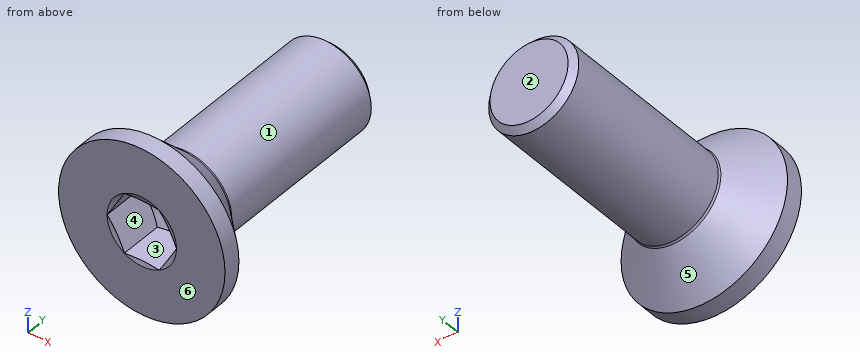
Solid Edge part; units mm, degrees
sketch "Sketch1" plane through (0, 0, 0) normal (0, 0, 1) x (1, 0, 0)
  line L0 (1.5, 0) -> (1.5, 6.14)
  line L1 (0, 6.14) -> (1.5, 6.14)
  line L2 (0, 0) -> (0, 6.14)
  line L3 (0, 0) -> (0, -1.86)
  line L4 (0, -1.86) -> (2.77, -1.86)
  line L5 (2.77, -1.86) -> (2.77, -1.27)
  line L6 (2.77, -1.27) -> (1.5, 0)
revolve "RevolvedProtrusion1" add sketch "Sketch1" angle 360 about axis through (0, 0, 0) along (0, 1, 0)
sketch "Sketch2" plane through (0, 0, 0) normal (1, 0, 0) x (0, 1, 0)
  line L0 (-1.86, 1.6515) -> (-0.76, 1.6515)
  line L1 (0.1935, 0) -> (-0.76, 1.6515)
  line L2 (-1.86, 0) -> (0.1935, 0)
  line L3 (-1.86, 0) -> (-1.86, 1.6515)
revolve "RevolvedCutout1" cut sketch "Sketch2" angle 360 about axis through (0, -4.5, 0) along (0, 1, 0)
sketch "Sketch3" plane through (0, -1.86, 0) normal (0, -1, 0) x (0, 0, 1)
  circle A0 centre (0, 0) radius 1.6515
  line L0 (-1, -0.5774) -> (0, -1.1547)
  line L1 (0, -1.1547) -> (1, -0.5774)
  line L2 (1, -0.5774) -> (1, 0.5774)
  line L3 (1, 0.5774) -> (0, 1.1547)
  line L4 (0, 1.1547) -> (-1, 0.5774)
  line L5 (-1, 0.5774) -> (-1, -0.5774)
extrude "Protrusion1" add sketch "Sketch3" against normal up to next
sketch "Sketch4" plane through (0, 0, 0) normal (0, 0, 1) x (1, 0, 0)
  line L0 (-1.1547, -1.86) -> (0, -1.86)
  line L1 (0, -1.86) -> (0, -1.5506)
  line L2 (0, -1.5506) -> (-1.1547, -1.86)
revolve "RevolvedCutout2" cut sketch "Sketch4" angle 360 about axis through (0, -4.5, 0) along (0, 1, 0)
fillet "Round1" radius 0.1 1 edges at (0, 0, -1.5)
chamfer "倒斜角_2" distance 0.2 angle 45 1 edges at (0, 6.14, -1.5)
cosmetic_thread "Thread1"
Could you check a few things on this model? Use its own coordinates, in mm. Face numbers are marked on the shaded views. A direction names the side the tool comes from. Round coordinates to 2 decimals unless told otherwise and drop trailing zeros. Write each loop counter-clockwise with the first axis right and the second up, starting at its lowest first coordinate (ties: lowest second). Pieces come first, ordered by that corner, then holes.
(1) Thinking about a two-plate mould opening in Z: for the marked faces 4, 5 and 6, which applies, +Z half, -Z half, draft (parallel to the pull), parting line (faces both ways), or undercut?
Findings below:
face 4: undercut
face 5: parting line
face 6: draft
(2) Suppose I cut it at A-A on y = 5. Write out the boundary of the cut face in (x, z).
Findings below:
outline: circle Ø3 at (0, 0)
(3) Which directions (+Z, -Z, +X, -X, +Y, -Y) give clear straight access to the entire face, cutting with the end or side of a thin tool? Please do the marked faces 1, 2 and 3.
Findings below:
face 1: +Y
face 2: +Z, -Z, +X, -X, +Y
face 3: -Y
(4) If I drill on probe 1 along Z at (x, y) = (0, 1.75); probe 2 along Z at (x, y) = (-0.85, -0.5); probe 3 along X at (y, z) = (3.75, -0.75), over which ranges is the centre line in solid material (lowest first)?
Findings below:
probe 1: z = -1.5 to 1.5
probe 2: z = -1.81 to -0.53, 0.53 to 1.81
probe 3: x = -1.3 to 1.3
(5) For pin 1 (1 mm diameter, centred on y = 2.5, z = -1, fed in from +X); pin 2 (0.6 mm diameter, centred on x = 0, y = -1, fed in from +Z); pin 3 (1 mm diameter, centred on x = 0, y = 2, fed in from -Z); pin 4 (2 mm diameter, centred on x = 0, y = 1.5, fed in from +Z), each with a flat end and sliding along its axis, tell me the tip position at first contact or that it passes through.
Findings below:
pin 1: stops at x = 1.41
pin 2: stops at z = 2.77
pin 3: stops at z = -1.5
pin 4: stops at z = 1.5
